The model under review builds one solid part; all positions refer to its coordinate system, in mm. A direction names the side the tool comes from. Round coordinates to 2 decimals unless told otherwise and drop trailing zeros. Order: outer loops, then holes, each group sorted by start corner. A loop starts at its lowest first (then second) coordinate and runs counter-clockwise, first axis right, second up. Notation, with made-up numbers: M 11,3 L 49,3 A13 cw 49,19 Z; hole C 1,-15 d11. An arc over 180 degrees is marked long. Use a Markdown table: item, result. Add a question column.
1. To check wall thickness, follow probe 1 along Z at (x, y) = (-2, 7.75); probe 2 along Z at (x, y) = (4.5, 2); probe 3 along Y at (x, z) = (-14, 35). State the ranges of each line that lie inside material, in increasing order.
2. Insertion check: P1, Ø6, axis at y = 10, z = -15, coming from the -X side; P2, Ø9, axis at x = 0, z = -62.5, coming from the -Y side; P3, Ø6, axis at y = 18, z = -43.5, coming from the +X side; P4, Ø5, axis at y = 14.5, z = -40.5, coming from the -X side. Each pin has a flat end and moves straight along its axis. Give the tip position at first contact, or say it passes through.
3. Consider section D-D on y = 12.75. Count the separate pieces of the cut face and the enclosed holes in it, then the cut area to 3 significant figures.
4. Consider section B-B on z = 0. State the section outline as (x, y) points, then the cut area to 4 significant figures.
5. Consider section A-A on x = 0. State the section outline as (y, z) points, then the cut area to 4 significant figures.
6. Consider section C-C on x = -18. State the section outline as (y, z) points.
7. The part is to be moulded in two halves that separate along Z. For faces 4 (the cylindrical face through (-17.34, 3.3, 78.1)), 5 (the flat face through (59, 6.5, 53)), 6 (the cylindrical face through (66.27, 9.86, -1.96)), say which applies: +Z half, -Z half, draft (parallel to the pull), parting line (faces both ways), or undercut.
8. For faces 1 (the cylindrical face through (-8.67, 3.45, -39.05)), 2 (the cylindrical face through (-0.651, 9.86, -57.543)), 3 (the cylindrical face through (-58.23, 13.34, -53.39)), list the 3-axis set-ups (+Z, -Z, +X, -X, +Y, -Y) from which the entire face can be reached by the end or side of a thin tool; tool diameter is ignored.
from build123d import *

# Parameters (mm, degrees)
SCHIZZO2_R                  = 28
TAGLIO_ESTRUSIONE1_DEPTH    = 21
RIPETIZIONECIRCOLARE1_COUNT = 6
SCHIZZO5_R                  = 5
TAGLIO_ESTRUSIONE2_DEPTH    = 21
SCHIZZO6_R                  = 40
TAGLIO_ESTRUSIONE3_DEPTH    = 7


with BuildPart() as part:
    # Schizzo1 → Rivoluzione1 (revolve)
    with BuildSketch(Plane.XY):
        Polygon((0, 0), (80, 0), (80, 6.5), (79, 6.5), (79, 20), (0, 20), align=None)
    revolve(axis=Axis((0, 0, 0), (0, 1, 0)))

    # Schizzo2 → Taglio-Estrusione1 (cut, through all)
    with BuildSketch(Plane.XZ):
        Circle(SCHIZZO2_R)
    extrude(amount=-TAGLIO_ESTRUSIONE1_DEPTH, mode=Mode.SUBTRACT)

    # Schizzo3 → M10 Foro filettato profondo1 (revolve, cut)
    with BuildSketch(Plane(origin=(62.5, 0, 0), x_dir=(0, 0, -1), z_dir=(1, 0, 0))):
        Polygon((0, 0), (0, 27.553657631), (4.25, 25), (4.25, 0), align=None)
    m10_foro_filettato_profondo1 = revolve(axis=Axis((62.5, -6.35, 0), (0, 1, 0)), mode=Mode.SUBTRACT)

    # RipetizioneCircolare1: M10 Foro filettato profondo1 ×6 about axis
    ripetizionecircolare1_axis = Axis((0, 0, 0), (0, 1, 0))
    for i in range(1, RIPETIZIONECIRCOLARE1_COUNT):
        add(m10_foro_filettato_profondo1.rotate(ripetizionecircolare1_axis, i * 360 / RIPETIZIONECIRCOLARE1_COUNT), mode=Mode.SUBTRACT)

    # Schizzo5 → Taglio-Estrusione2 (cut, through all)
    with BuildSketch(Plane.XZ):
        with Locations((0, 62.5)):
            Circle(SCHIZZO5_R)
        with Locations((0, -62.5)):
            Circle(SCHIZZO5_R)
    extrude(amount=-TAGLIO_ESTRUSIONE2_DEPTH, mode=Mode.SUBTRACT)

    # Schizzo6 → Taglio-Estrusione3 (cut)
    with BuildSketch(Plane.XZ):
        Circle(SCHIZZO6_R)
    extrude(amount=-TAGLIO_ESTRUSIONE3_DEPTH, mode=Mode.SUBTRACT)


solid = part.part
Answer block:
| question | item | result |
|---|---|---|
| 1 | probe 1 | -78.97 to -67.08, -57.92 to -27.93, 27.93 to 57.92, 67.08 to 78.97 |
| 1 | probe 2 | -79.87 to -64.68, -60.32 to -39.75, 39.75 to 60.32, 64.68 to 79.87 |
| 1 | probe 3 | 7 to 20 |
| 2 | P1 | x = -78.08 |
| 2 | P2 | through |
| 2 | P3 | x = 67.83 |
| 2 | P4 | x = -69.26 |
| 3 | separate pieces | 1 |
| 3 | enclosed holes | 9 |
| 3 | area | 16,600 mm^2 |
| 4 | outline | M -80,0 L -66.75,0 L -66.75,20 L -79,20 L -79,6.5 L -80,6.5 Z; M -58.25,0 L -40,0 L -40,7 L -28,7 L -28,20 L -58.25,20 Z; M 28,7 L 40,7 L 40,0 L 58.25,0 L 58.25,20 L 28,20 Z; M 66.75,0 L 80,0 L 80,6.5 L 79,6.5 L 79,20 L 66.75,20 Z |
| 4 | area | 1,545 mm^2 |
| 5 | outline | M 0,-80 L 6.5,-80 L 6.5,-79 L 20,-79 L 20,-67.5 L 0,-67.5 Z; M 0,-57.5 L 20,-57.5 L 20,-28 L 7,-28 L 7,-40 L 0,-40 Z; M 0,40 L 7,40 L 7,28 L 20,28 L 20,57.5 L 0,57.5 Z; M 0,67.5 L 20,67.5 L 20,79 L 6.5,79 L 6.5,80 L 0,80 Z |
| 5 | area | 1,485 mm^2 |
| 6 | outline | M 0,-77.95 L 6.5,-77.95 L 6.5,-76.92 L 20,-76.92 L 20,-21.45 L 7,-21.45 L 7,-35.72 L 0,-35.72 Z; M 0,35.72 L 7,35.72 L 7,21.45 L 20,21.45 L 20,76.92 L 6.5,76.92 L 6.5,77.95 L 0,77.95 Z |
| 7 | face 4 | parting line |
| 7 | face 5 | draft |
| 7 | face 6 | undercut |
| 8 | face 1 | -Y |
| 8 | face 2 | +Y, -Y |
| 8 | face 3 | +Y |
